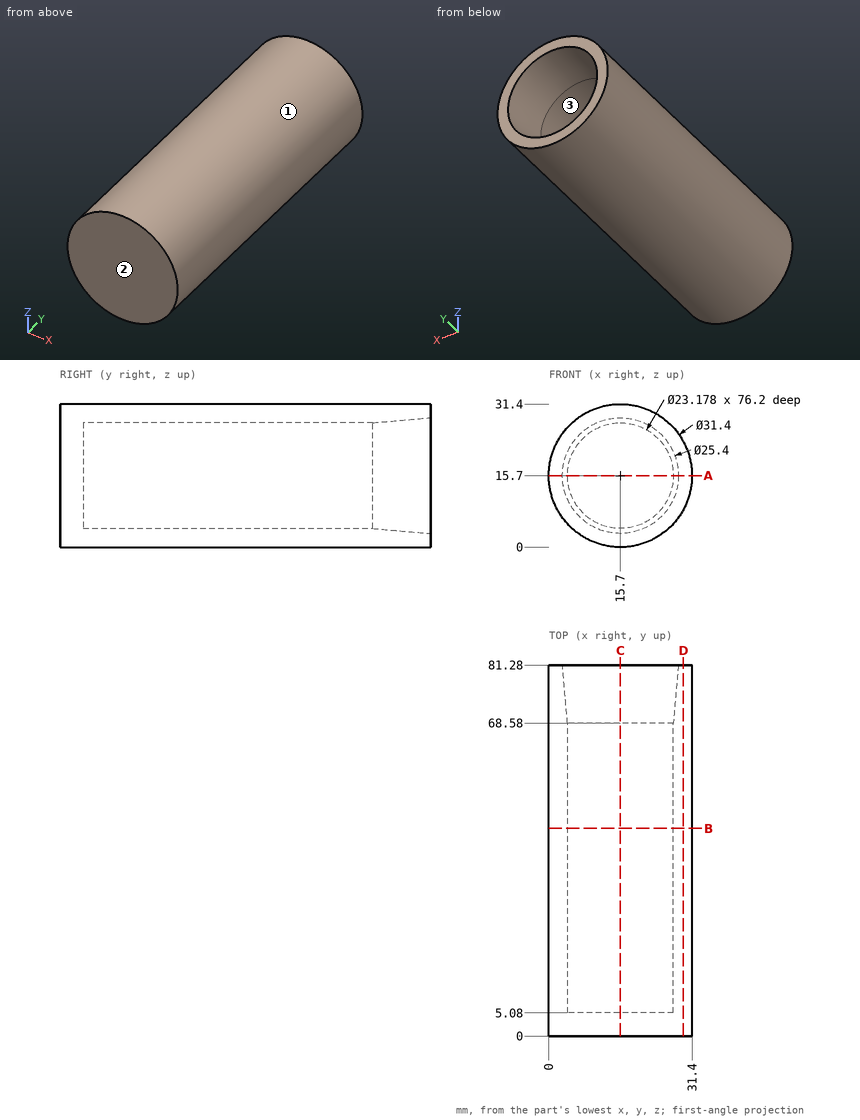
Source: three-view drawing plus pictorial views. Frame: mm from the lowest corner of the part. Round coordinates to 2 decimals unless told otherwise and drop trailing zeros. Loops run counter-clockwise (first coordinate to the right, second up) from the corner with the lowest first, then second, coordinate; pieces in that order, holes last. Notation, with made-up numbers: M -17,12 L 0,12 A15 cw 0,29 Z; hole C 41.25,-18.5 d11. An arc over 180 degrees is marked long. Put each result on its own line as item: value. Start each with the question number.
(1) Section query C-C (x = 15.7). Return loops of the section in (y, z).
(2) Material intervals for line 1 along X through (y, z) = (53.5, 15.7); line 2 along X through (y, z) = (18.5, 13.5) (1 decimal); line 3 along Z through (x, y) = (21.5, 50), sorted ascending. Write a range as [from, to].
(3) Section query D-D (x = 29.5). Return loops of the section in (y, z), then the cut area to 3 significant figures.
(4) Draft query along Z for the marked faces 1, 2 and 3. Return one class per face: +Z half, -Z half, draft (parallel to the pull), parting line (faces both ways), or undercut.
(5) Section query A-A (z = 15.7). Return loops of the section in (x, y).
(6) Section query B-B (y = 45.5). Return loops of the section in (x, z).
(7) Contact query for flat-ended pins moving along their axis: pin 1 Ø4 at (y, z) = (51.5, 21.5) entering from -X; pin 2 Ø1 at (x, y) = (19.5, 29.5) entering from +Z; pin 3 Ø10 at (x, y) = (11, 15) entering from -Z; pin 4 Ø8 at (x, y) = (8.5, 40.5) entering from -Z. Output: stop coordinate, or through.
Findings below:
1. outline: M 0,0 L 81.28,0 L 81.28,3 L 68.58,4.11 L 5.08,4.11 L 5.08,27.29 L 68.58,27.29 L 81.28,28.4 L 81.28,31.4 L 0,31.4 Z
2. line 1: x = [0, 4.11], [27.29, 31.4]
2. line 2: x = [0.2, 4.3], [27.1, 31.2]
2. line 3: z = [1.11, 5.67], [25.73, 30.29]
3. outline: M 0,8.21 L 81.28,8.21 L 81.28,23.19 L 0,23.19 Z
3. area: 1,220 mm2
4. face 1: parting line
4. face 2: draft
4. face 3: undercut
5. outline: M 0,0 L 31.4,0 L 31.4,81.28 L 28.4,81.28 L 27.29,68.58 L 27.29,5.08 L 4.11,5.08 L 4.11,68.58 L 3,81.28 L 0,81.28 Z
6. outline: C 15.7,15.7 d31.4; hole C 15.7,15.7 d23.18
7. pin 1: stops at x = 0.47
7. pin 2: stops at z = 31.05
7. pin 3: stops at z = 0
7. pin 4: stops at z = 0.33
